For this review, use the dimensioned drawing (mm, ordinates from the lowest corner) and the shaded views. A direction names the side the tool comes from. Give positions to 0.01 mm unless a question says otherwise; leave off trailing zeros. Loops run counter-clockwise (first coordinate to the right, second up) from the corner with the lowest first, then second, coordinate; pieces in that order, holes last. Notation, with made-up numbers: M -15.75,-1 L -8.75,-1 A17 ccw -8.75,26 Z; hole C -13.75,-26.75 d11. An arc over 180 degrees is marked long. Use a Markdown table: item, result. Add a question column.
(1) Add section D-D, the plane x = 13.75. Give the boundary of the cut face in (y, z), then the cut area to 3 significant figures.
(2) For probe 1 along Y at (x, z) = (10, 11); probe 2 along Z at (x, y) = (16.25, 17.25); probe 3 along X at (y, z) = (18.5, 8.25), list the stretches that pass through material, from the lowest coordinate up.
(3) Insertion check: pin 1 Ø1.5 at (x, z) = (11, 1) entering from +Y; pin 2 Ø0.9 at (y, z) = (4, 1) entering from -X; pin 3 Ø1.5 at (y, z) = (2.5, 1) entering from +X. Each pin has a flat end and moves straight along its axis. Give the tip position at first contact, or say it passes through.
(4) Add section B-B, the plane y = 20. Give the boundary of the cut face in (x, z), then the cut area to 3 significant figures.
(5) Add section C-C, the plane z = 6. Give the boundary of the cut face in (x, y).
(6) Draft analysis for pull direction Y (two halves, no side actions). For the marked faces 3, 4 and 5, state which applies: pulls with the +Y half, pulls with the -Y half, needs draft (parallel to the pull), parting line crosses it, or undercut.
(7) Add section A-A, the plane x = 10. Give the boundary of the cut face in (y, z).
(8) For the marked faces 1 and 2, list the 3-axis set-ups (+Z, -Z, +X, -X, +Y, -Y) from which the entire face can be reached by the end or side of a thin tool; tool diameter is ignored.
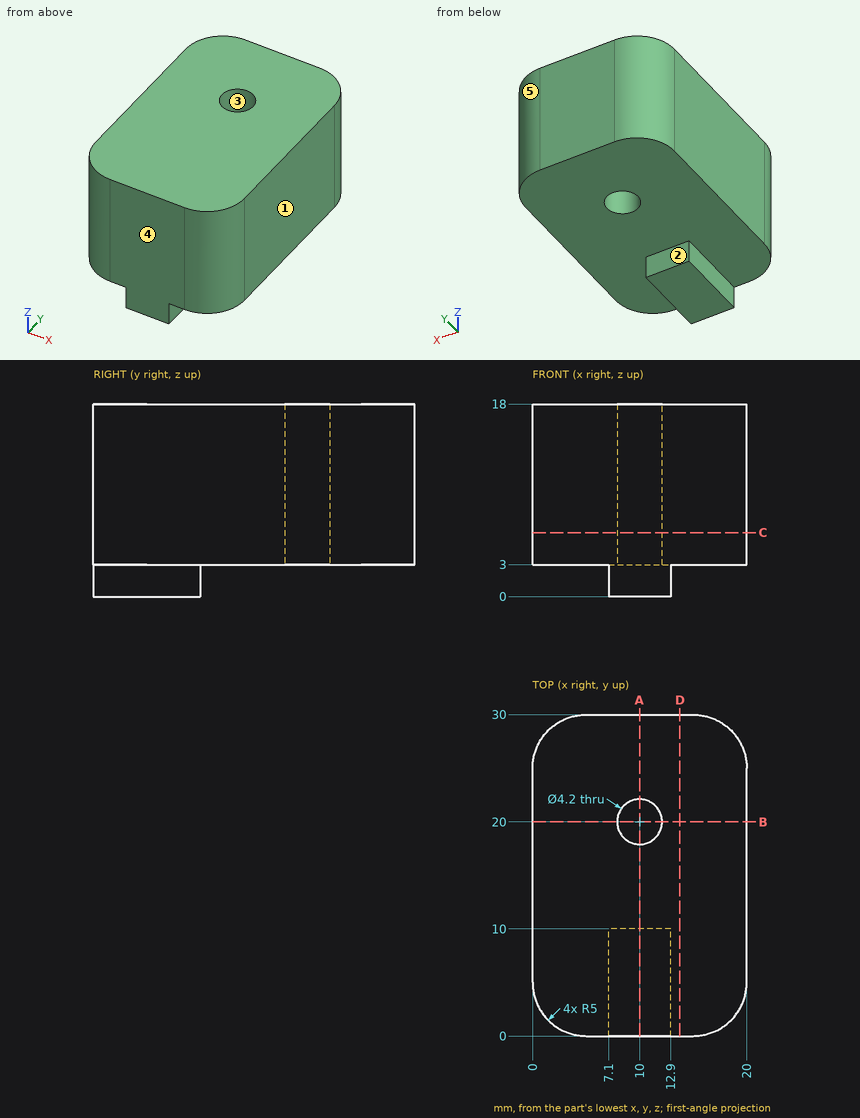
Established:
| question | item | result |
|---|---|---|
| 1 | outline | M 0,3 L 30,3 L 30,18 L 0,18 Z |
| 1 | area | 450 mm^2 |
| 2 | probe 1 | 0 to 17.9, 22.1 to 30 |
| 2 | probe 2 | 3 to 18 |
| 2 | probe 3 | 0 to 8.53, 11.47 to 20 |
| 3 | pin 1 | y = 10 |
| 3 | pin 2 | x = 7.1 |
| 3 | pin 3 | x = 12.9 |
| 4 | outline | M 0,3 L 7.9,3 L 7.9,18 L 0,18 Z; M 12.1,3 L 20,3 L 20,18 L 12.1,18 Z |
| 4 | area | 237 mm^2 |
| 5 | outline | M 0,5 A5 ccw 5,0 L 15,0 A5 ccw 20,5 L 20,25 A5 ccw 15,30 L 5,30 A5 ccw 0,25 Z; hole C 10,20 d4.2 |
| 6 | face 3 | undercut |
| 6 | face 4 | pulls with the -Y half |
| 6 | face 5 | pulls with the +Y half |
| 7 | outline | M 0,0 L 10,0 L 10,3 L 17.9,3 L 17.9,18 L 0,18 Z; M 22.1,3 L 30,3 L 30,18 L 22.1,18 Z |
| 8 | face 1 | +Z, -Z, +X, +Y, -Y |
| 8 | face 2 | -Z, +X, -X, +Y |
